from build123d import *

# Parameters (mm, degrees)
ESQUISSE1_W             = 35
ESQUISSE1_H             = 20
ESQUISSE1_W_2           = 32
ESQUISSE1_H_2           = 17
BOSS_EXTRU_1_DEPTH      = 600
ENL_V_MAT_EXTRU_1_DEPTH = 602.352641966
ENL_V_MAT_EXTRU_3_DEPTH = 602.352641966


with BuildPart() as part:
    # Esquisse1 → Boss.-Extru.1 (new body)
    with BuildSketch(Plane.XY):
        with Locations((17.5, 10)):
            Rectangle(ESQUISSE1_W, ESQUISSE1_H)
        with Locations((17.5, 10)):
            Rectangle(ESQUISSE1_W_2, ESQUISSE1_H_2, mode=Mode.SUBTRACT)
    extrude(amount=BOSS_EXTRU_1_DEPTH)

    # Esquisse2 → Enlèv. mat.-Extru.1 (cut, through all)
    with BuildSketch(Plane(origin=(0, 0, 0), x_dir=(1, 0, 0), z_dir=(0, 1, 0))):
        Polygon((0, -600), (35, -565), (35, -600), align=None)
    extrude(amount=ENL_V_MAT_EXTRU_1_DEPTH, mode=Mode.SUBTRACT)

    # Esquisse4 → Enlèv. mat.-Extru.3 (cut, through all)
    with BuildSketch(Plane(origin=(0, 0, 0), x_dir=(1, 0, 0), z_dir=(0, 1, 0))):
        Polygon((0, 0), (35, -35), (35, 0), align=None)
    extrude(amount=ENL_V_MAT_EXTRU_3_DEPTH, mode=Mode.SUBTRACT)


solid = part.part
Build history of the part. All positions in model axes, mm. A direction names the side the tool comes from. Coordinates: 2 decimals unless noted, no trailing zeros. Write each loop counter-clockwise with the first axis right and the second up, starting at its lowest first coordinate (ties: lowest second). Pieces come first, ordered by that corner, then holes. Notation, with made-up numbers: (32, -8) -> (43, -8) arc R20 ccw to (43, -2) -> close; hole circle Ø3 at (81.25, -13). An arc over 180 degrees is marked (long way). Use CSV: the item, a comma, the result in double quotes. Start each with the question number.
Q1. Drill centre lines: probe 1 along Y at (x, z) = (15, 79.5); probe 2 along X at (y, z) = (17, 441.5); probe 3 along Z at (x, y) = (27, 18.75). Where is each one in solid material? Low to high.
Q2. Cut at C-C, the plane z = 523. List the corners of the cut face in (x, y).
Q3. Cut at A-A, the plane x = 24. List the corners of the cut face in (y, z).
Q4. 3-axis set-ups, long thin cutter, end or side, ignore diameter. For faces 1 (the flat face through (17, 20, 296)), 2 (the flat face through (17, 18.5, 296)): which of +Z, -Z, +X, -X, +Y, -Y reach the whole face in a straight line?
Q5. Pull direction Y, two halves, no side cores. Call faces 3 (the flat face through (17, 0, 296)), 4 (the flat face through (1.5, 10, 296)), 5 (the flat face through (16, 19, 16)): released by +Y, released by -Y, zero draft, split by the parting line, or undercut.
Q6. Cut at B-B, the plane y = 13.25. List the corners of the cut face in (x, z).
Q7. Flat gauge pins, fed straight in: pin 1 Ø8.5 at (y, z) = (11.5, 339) entering from -X; pin 2 Ø8 at (x, y) = (17.5, 15) entering from -Z; pin 3 Ø6 at (x, y) = (14, 3) entering from -Z. Where does each tip first touch, or does it go through?
Checked values:
1,probe 1,"y = 0 to 1.5, 18.5 to 20"
1,probe 2,"x = 0 to 1.5, 33.5 to 35"
1,probe 3,"z = 27 to 573"
2,outline,"(0, 0) -> (35, 0) -> (35, 20) -> (0, 20) -> close; hole (1.5, 1.5) -> (33.5, 1.5) -> (33.5, 18.5) -> (1.5, 18.5) -> close"
3,outline,"(0, 24) -> (1.5, 24) -> (1.5, 576) -> (0, 576) -> close; (18.5, 24) -> (20, 24) -> (20, 576) -> (18.5, 576) -> close"
4,face 1,"+Z, -Z, +X, -X, +Y"
4,face 2,"+Z, -Z"
5,face 3,"released by -Y"
5,face 4,"undercut"
5,face 5,"zero draft"
6,outline,"(0, 0) -> (1.5, 1.5) -> (1.5, 598.5) -> (0, 600) -> close; (33.5, 33.5) -> (35, 35) -> (35, 565) -> (33.5, 566.5) -> close"
7,pin 1,"stops at x = 0"
7,pin 2,"stops at z = 15.56"
7,pin 3,"stops at z = 11.4"
